Can you work these out from the model? Positions are in its coordinate system, mm. Face numbers are marked on the shaded views. A direction names the side the tool comes from. Give positions to 0.01 mm unless a question says otherwise; leave off trailing zeros. Order: outer loops, then holes, each group sorted by start corner. A loop starts at its lowest first (then second) coordinate and runs counter-clockwise, first axis right, second up. Notation, with made-up numbers: (14, 52.25) -> (60, 52.25) arc R25 ccw to (60, 75.25) -> close; hole circle Ø2 at (24.5, 60.25). An arc over 180 degrees is marked (long way). Answer as a JSON object with one key per item and string values.
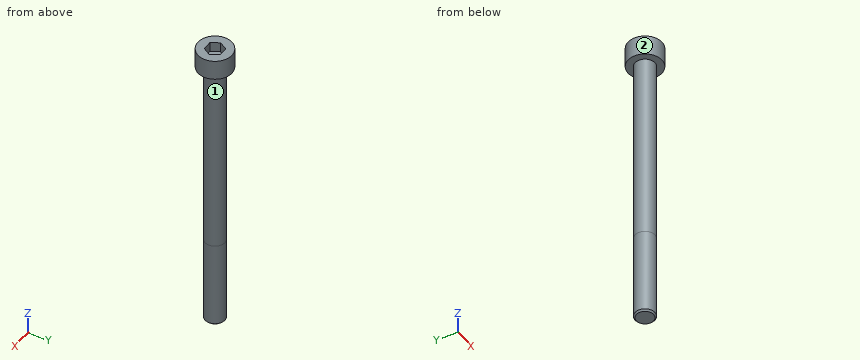
Solid Edge part; units mm, degrees
sketch "Sketch1" plane through (0, 0, 0) normal (0, 0, 1) x (1, 0, 0)
  circle A0 centre (0, 0) radius 4.25
extrude "Protrusion1" add sketch "Sketch1" along normal blind 5
sketch "Sketch2" plane through (0, 0, 0) normal (0, 0, -1) x (1, 0, 0)
  circle A0 centre (0, 0) radius 2.5
extrude "Protrusion2" add sketch "Sketch2" along normal blind 70
sketch "Sketch3" plane through (0, 0, -70) normal (0, 0, -1) x (1, 0, 0)
  circle A0 centre (0, 0) radius 2.4997
extrude "Cutout1" cut sketch "Sketch3" against normal blind 22 flip side to cut
chamfer "Chamfer_1" distance 0.375 angle 45 1 edges at (-2.4997, 0, -70)
sketch "Sketch4" plane through (0, 0, 5) normal (0, 0, 1) x (1, 0, 0)
  line L0 (-1.1547, 2) -> (1.1547, 2)
  line L1 (2.3094, 0) -> (1.1547, 2)
  line L2 (1.1547, -2) -> (2.3094, 0)
  line L3 (-1.1547, -2) -> (1.1547, -2)
  line L4 (-2.3094, 0) -> (-1.1547, -2)
  line L5 (-1.1547, 2) -> (-2.3094, 0)
extrude "Cutout2" cut sketch "Sketch4" against normal blind 2.5
properties part number "300282"
1. Please list where these lines run through material, in increasing order: L1, parallel to Z at x = 1, y = 1; L2, parallel to Y at x = 1.5, z = -3; L3, parallel to X at y = -0.25, z = -54.
Worked answers:
{"L1": "-70 to 2.5", "L2": "-2 to 2", "L3": "-2.49 to 2.49"}
2. Will these pins go through, and if not, where does the flat tip stop? pin 1 Ø1.5 at (y, z) = (-3, -23.5) entering from -X; pin 2 Ø1.5 at (x, z) = (1, -29) entering from +Y; pin 3 Ø3 at (x, z) = (-2, -18.5) entering from -Y.
Worked answers:
{"pin 1": "x = -1.09", "pin 2": "y = 2.49", "pin 3": "y = -2.45"}
3. If we section it at B-B on z = -56.5: Please give me the cut outline in (x, y), then the cut area to 3 significant figures.
Worked answers:
{"outline": "circle Ø5 at (0, 0)", "area": "19.6 mm²"}
4. If we section it at C-C on y = -3.5: Please give me the cut outline in (x, z), then the cut area to 3 significant figures.
Worked answers:
{"outline": "(-2.41, 0) -> (2.41, 0) -> (2.41, 5) -> (-2.41, 5) -> close", "area": "24.1 mm²"}
5. For the marked faces 1 and 2, which set-ups out of +Z, -Z, +X, -X, +Y, -Y let a thin tool reach every point of the face, with its end or its side?
Worked answers:
{"face 1": "-Z", "face 2": "+Z, -Z"}
